Verification items for the finished model (mm, model axes). A direction names the side the tool comes from. Coordinates: 2 decimals unless noted, no trailing zeros. Write each loop counter-clockwise with the first axis right and the second up, starting at its lowest first coordinate (ties: lowest second). Pieces come first, ordered by that corner, then holes.
Autodesk Inventor part; units mm, degrees
ref_plane "YZ Plane" through (0, 0, 0) normal (1, 0, 0) x (0, 1, 0)
ref_plane "XZ Plane" through (0, 0, 0) normal (0, 1, 0) x (-1, 0, 0)
ref_plane "XY Plane" through (0, 0, 0) normal (0, 0, 1) x (1, 0, 0)
sketch "Sketch1" plane through (0, 0, 0) normal (0, 1, 0) x (-1, 0, 0)
  line L0 (-34, 0) -> (-34, -8)
  line L1 (-34, -8) -> (0, -8)
  line L2 (0, -8) -> (0, 0)
  line L3 (0, 0) -> (0, -1)
  line L4 (-33, -1) -> (-33, -7)
  line L5 (-33, -7) -> (-1, -7)
  line L6 (-1, -7) -> (-1, -1)
  line L7 (-5, 0) -> (-5, 10)
  line L8 (-5, 10) -> (-29, 10)
  line L9 (-29, 10) -> (-29, 0)
  line L10 (-29, 10) -> (-29, 9)
  line L11 (-1, -1) -> (-5, -1)
  line L12 (-29, -1) -> (-33, -1)
  line L13 (-29, -1) -> (-28, -1)
  line L14 (0, 0) -> (-5, 0)
  line L15 (-34, 0) -> (-29, 0)
  line L16 (-28, -1) -> (-28, 9)
  line L17 (-28, 9) -> (-6, 9)
  line L18 (-6, 9) -> (-6, -1)
  line L19 (-6, -1) -> (-5, -1)
  line L20 (0, 0) -> (-5, 0)
  dimension "d0" = 34
  dimension "d1" = 8
  dimension "d4" = 32
  dimension "d5" = 6
  dimension "d9" = 24
  dimension "d17" = 10
  dimension "d18" = 22
extrude "Extrusion1" add sketch "Sketch1" along normal blind 3
sketch "Sketch2" plane through (0, 3, 0) normal (0, 1, 0) x (1, 0, 0)
  line L0 (0, 8) -> (0, 0)
  line L1 (34, 8) -> (0, 8)
  line L2 (34, 0) -> (34, 8)
  line L3 (29, 0) -> (34, 0)
  line L4 (29, -10) -> (29, 0)
  line L5 (5, -10) -> (29, -10)
  line L6 (5, 0) -> (5, -10)
  line L7 (0, 0) -> (5, 0)
extrude "Extrusion2" add sketch "Sketch2" along normal blind 1
sketch "Sketch3" plane through (0, 3, 0) normal (0, -1, 0) x (1, 0, 0)
  line L0 (33, -7) -> (33, -1)
  line L1 (33, -1) -> (28, -1)
  line L2 (28, -1) -> (28, 9)
  line L3 (28, 9) -> (6, 9)
  line L4 (6, 9) -> (6, -1)
  line L5 (6, -1) -> (1, -1)
  line L6 (1, -1) -> (1, -7)
  line L7 (1, -7) -> (33, -7)
  line L8 (28, 9) -> (6, 9)
  line L9 (6, 9) -> (6, 8)
  line L10 (6, 9) -> (6, -1)
  line L11 (6, 8) -> (7, 8)
  line L12 (7, 8) -> (8.5, 8)
  line L13 (8.5, 8) -> (8.5, 2)
  line L14 (8.5, 2) -> (7, 2)
  line L15 (7, 2) -> (7, 8)
  line L16 (7, 2) -> (7, 1)
  line L17 (7, 1) -> (8.5, 1)
  line L18 (8.5, 1) -> (8.5, -5)
  line L19 (8.5, -5) -> (7, -5)
  line L20 (7, -5) -> (7, 1)
  line L21 (28, -1) -> (28, 9)
  line L22 (28, 9) -> (28, 8)
  line L23 (28, 8) -> (27, 8)
  line L24 (27, 8) -> (25.5, 8)
  line L25 (25.5, 8) -> (25.5, 2)
  line L26 (25.5, 2) -> (27, 2)
  line L27 (27, 2) -> (27, 8)
  line L28 (27, 2) -> (27, 1)
  line L29 (27, 1) -> (25.5, 1)
  line L30 (25.5, 1) -> (25.5, -5)
  line L31 (25.5, -5) -> (27, -5)
  line L32 (27, -5) -> (27, 1)
  point P0 (0, 0)
  dimension "d23" = 1
  dimension "d24" = 1
  dimension "d26" = 1.5
  dimension "d27" = 6
  dimension "d28" = 1
  dimension "d29" = 1.5
  dimension "d30" = 6
  dimension "d31" = 1
  dimension "d32" = 1
  dimension "d33" = 1.5
  dimension "d34" = 6
  dimension "d35" = 1
extrude "Extrusion3" cut sketch "Sketch3" against normal blind 1 contours L32 L31 L30 L29 | L27 L26 L25 L24 | L17 L18 L19 L20 | L12 L13 L14 L15
sketch "Sketch4" plane through (0, 0, 0) normal (0, -1, 0) x (1, 0, 0)
  point P0 (0, 0)
properties part number "led-reed-compartment"
1. Sectioned sample at C-C, the plane x = 13. Record the boundary of the cut face in (y, z), and give its area (3 significant figures).
2. Gauge pin test, flat end, axial feed: P1, Ø1.1, axis at y = 3.5, z = 4.5, coming from the +X side. Record the tip position at first contact, or that the pin passes through.
3. Material ranges on L1, parallel to X at y = 3.3, z = 0.75; L2, parallel to X at y = 3.2, z = -1.75; L3, parallel to Z at x = 26.5, y = 2.5, recorded low to high.
4. Sectioned sample at B-B, the plane y = 2.2. Record the boundary of the cut face in (x, z).
5. Draft check along Z on faces 6 (the flat face through (0, 2, -4)), 7 (the flat face through (2, 2, 0)), 8 (the flat face through (17, 1, 9)), 9 (the flat face through (26.3, 3.5, 1)). Enter one of: pulls with the +Z half, pulls with the -Z half, needs draft (parallel to the pull), parting line crosses it, or undercut.
6. Sectioned sample at D-D, the plane z = -0.5. Record the boundary of the cut face in (x, y), and give its area (3 significant figures).
7. Sectioned sample at A-A, the plane z = -4.5. Record the boundary of the cut face in (x, y), and give its area (3 significant figures).
8. Tool access check on faces 1 (the flat face through (17, 4, 1)), 2 (the flat face through (31, 1, -1)), 3 (the flat face through (7, 3.5, -2)), 4 (the flat face through (5, 2, 5)), 5 (the flat face through (29, 2, 5)). Record the directions out of +Z, -Z, +X, -X, +Y, -Y that give a thin tool (end or side, any length) a straight path to the whole face; none if there is none.
Outcome:
1. outline: (0, -8) - (4, -8) - (4, 10) - (0, 10) - (0, 9) - (3, 9) - (3, -7) - (0, -7) - close
1. area: 24.0 mm2
2. P1: stops at x = 29
3. L1: x = 5 to 7, 8.5 to 25.5, 27 to 29
3. L2: x = 0 to 7, 8.5 to 25.5, 27 to 34
3. L3: z = -8 to -7, 9 to 10
4. outline: (0, -8) - (34, -8) - (34, 0) - (29, 0) - (29, 10) - (5, 10) - (5, 0) - (0, 0) - close; hole (1, -7) - (33, -7) - (33, -1) - (28, -1) - (28, 9) - (6, 9) - (6, -1) - (1, -1) - close
5. face 6: needs draft
5. face 7: pulls with the +Z half
5. face 8: undercut
5. face 9: undercut
6. outline: (0, 0) - (6, 0) - (6, 3) - (7, 3) - (7, 4) - (0, 4) - close; (8.5, 3) - (25.5, 3) - (25.5, 4) - (8.5, 4) - close; (27, 3) - (28, 3) - (28, 0) - (34, 0) - (34, 4) - (27, 4) - close
6. area: 67.0 mm2
7. outline: (0, 0) - (1, 0) - (1, 3) - (7, 3) - (7, 4) - (0, 4) - close; (8.5, 3) - (25.5, 3) - (25.5, 4) - (8.5, 4) - close; (27, 3) - (33, 3) - (33, 0) - (34, 0) - (34, 4) - (27, 4) - close
7. area: 37.0 mm2
8. face 1: +Z, -Z, +X, -X, +Y
8. face 2: -Y
8. face 3: +Y, -Y
8. face 4: +Z, -X, +Y, -Y
8. face 5: +Z, +X, +Y, -Y
